Print and shaded views of the part. All mm, measured from the part's lowest x, y and z. Coordinates: 2 decimals unless noted, no trailing zeros. Loops run counter-clockwise (first coordinate to the right, second up) from the corner with the lowest first, then second, coordinate; pieces in that order, holes last. Notation, with made-up numbers: (-40, 42) -> (-16, 42) arc R30 cw to (-16, 68) -> close; hole circle Ø11 at (15.25, -2.5). An arc over 180 degrees is marked (long way). One line per question, with ' | ' between items. Start each with the question number.
1) Cut at D-D (z = 0.5). List the corners of the cut face in (x, y).
2) Drop a flat-ended pin along its axis: pin 1 (6 mm diameter, centred on x = 10, y = 9.32, fed in from +Z). Give the stop position or say it passes through.
3) Probe L1, parallel to Y at x = 30, z = 3.2; L2, parallel to X at y = 9.25, z = 3.9; L3, parallel to X at y = 7.75, z = 0.7. List the from-to ranges inside material, lowest first. Write a range as from..to.
4) Cut at C-C (y = 11). Count the separate pieces of the cut face and the enclosed holes in it, plus the area to 3 significant figures.
5) Cut at A-A (x = 30). List the corners of the cut face in (y, z).
6) Two-plate mould, pull along X, no slides. Class the marked faces 1, 2, 3 and 4: released by +X, released by -X, zero draft, split by the parting line, or undercut.
7) Cut at B-B (z = 4.4). List the corners of the cut face in (x, y).
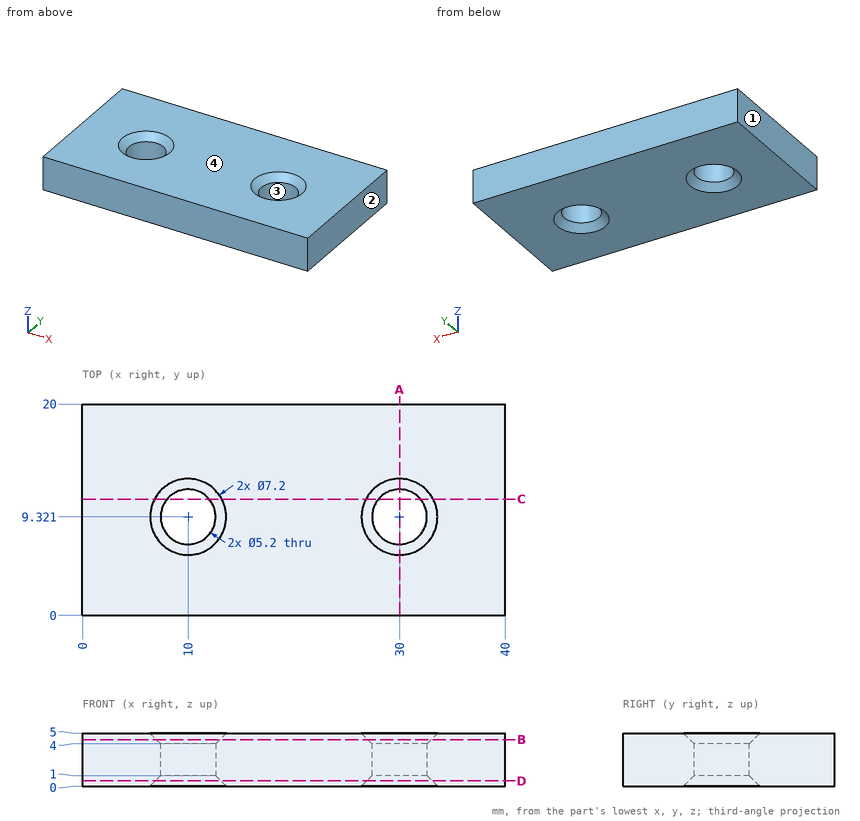
Reported:
1) outline: (0, 0) -> (40, 0) -> (40, 20) -> (0, 20) -> close; hole circle Ø6.2 at (10, 9.32); hole circle Ø6.2 at (30, 9.32)
2) pin 1: stops at z = 4.4
3) L1: y = 0..6.72, 11.92..20 | L2: x = 0..7.4, 12.6..27.4, 32.6..40 | L3: x = 0..7.56, 12.44..27.56, 32.44..40
4) separate pieces: 3 | enclosed holes: 0 | area: 155 mm²
5) outline: (0, 0) -> (5.72, 0) -> (6.72, 1) -> (6.72, 4) -> (5.72, 5) -> (0, 5) -> close; (11.92, 1) -> (12.92, 0) -> (20, 0) -> (20, 5) -> (12.92, 5) -> (11.92, 4) -> close
6) face 1: released by -X | face 2: released by +X | face 3: undercut | face 4: zero draft
7) outline: (0, 0) -> (40, 0) -> (40, 20) -> (0, 20) -> close; hole circle Ø6 at (10, 9.32); hole circle Ø6 at (30, 9.32)
